from build123d import *

# Parameters (mm, degrees)
F0_W      = 20
F0_H      = 20
F1_DEPTH  = 20
F2_R      = 2.6
F3_DEPTH  = 1
F4_R      = 2.6
F5_DEPTH  = 1
F6_R      = 2.6
F7_DEPTH  = 1
F8_R      = 2.6
F9_DEPTH  = 1
F10_R     = 2.6
F11_DEPTH = 1
F13_DEPTH = 1


with BuildPart() as f1:
    # F0 (on Front) → F1 (new body)
    with BuildSketch(Plane.XZ):
        with Locations((10, 10)):
            Rectangle(F0_W, F0_H)
    extrude(amount=F1_DEPTH)

    # F2 (on face) → F3 (cut)
    with BuildSketch(Plane.XZ.offset(20)):
        with Locations((10, 10)):
            Circle(F2_R)
        with Locations((5, 15)):
            Circle(F2_R)
        with Locations((15, 15)):
            Circle(F2_R)
        with Locations((15, 5)):
            Circle(F2_R)
        with Locations((5, 5)):
            Circle(F2_R)
    extrude(amount=-F3_DEPTH, mode=Mode.SUBTRACT)

    # F4 (on face) → F5 (cut)
    with BuildSketch(Plane(origin=(0, 0, 0), x_dir=(-1, 0, 0), z_dir=(0, 1, 0))):
        with Locations((-5, 15)):
            Circle(F4_R)
        with Locations((-15, 5)):
            Circle(F4_R)
    extrude(amount=-F5_DEPTH, mode=Mode.SUBTRACT)

    # F6 (on face) → F7 (cut)
    with BuildSketch(Plane(origin=(0, 0, 0), x_dir=(0, -1, 0), z_dir=(-1, 0, 0))):
        with Locations((10, 10)):
            Circle(F6_R)
        with Locations((15, 15)):
            Circle(F6_R)
        with Locations((5, 5)):
            Circle(F6_R)
    extrude(amount=-F7_DEPTH, mode=Mode.SUBTRACT)

    # F8 (on face) → F9 (cut)
    with BuildSketch(Plane.YZ.offset(20)):
        with Locations((-15, 5)):
            Circle(F8_R)
        with Locations((-15, 15)):
            Circle(F8_R)
        with Locations((-5, 15)):
            Circle(F8_R)
        with Locations((-5, 5)):
            Circle(F8_R)
    extrude(amount=-F9_DEPTH, mode=Mode.SUBTRACT)

    # F10 (on face) → F11 (cut)
    with BuildSketch(Plane(origin=(0, 0, 0), x_dir=(1, 0, 0), z_dir=(0, 0, -1))):
        with Locations((10, 10)):
            Circle(F10_R)
    extrude(amount=-F11_DEPTH, mode=Mode.SUBTRACT)

    # F12 (on face) → F13 (cut)
    with BuildSketch(Plane.XY.offset(20)):
        with BuildLine():
            ThreePointArc((4, -6.6), (5.838478, -5.838478), (6.6, -4))
            ThreePointArc((6.6, -4), (5.838478, -2.161522), (4, -1.4))
            ThreePointArc((4, -1.4), (1.4, -4), (4, -6.6))
        make_face()
        with BuildLine():
            ThreePointArc((6.6, -16), (5.838478, -14.161522), (4, -13.4))
            ThreePointArc((4, -13.4), (2.161522, -14.161522), (1.4, -16))
            ThreePointArc((1.4, -16), (4, -18.6), (6.6, -16))
        make_face()
        with BuildLine():
            ThreePointArc((6.6, -10), (5.838478, -8.161522), (4, -7.4))
            ThreePointArc((4, -7.4), (1.4, -10), (4, -12.6))
            ThreePointArc((4, -12.6), (5.838478, -11.838478), (6.6, -10))
        make_face()
        with BuildLine():
            Line((13.4, -16), (18.6, -16))
            ThreePointArc((18.6, -16), (17.838478, -14.161522), (16, -13.4))
            ThreePointArc((16, -13.4), (14.161522, -14.161522), (13.4, -16))
        make_face()
        with BuildLine():
            ThreePointArc((13.4, -4), (14.161522, -5.838478), (16, -6.6))
            ThreePointArc((16, -6.6), (17.838478, -5.838478), (18.6, -4))
            Line((18.6, -4), (13.4, -4))
        make_face()
        with BuildLine():
            ThreePointArc((16, -7.4), (13.4, -10), (16, -12.6))
            ThreePointArc((16, -12.6), (17.838478, -11.838478), (18.6, -10))
            ThreePointArc((18.6, -10), (17.838478, -8.161522), (16, -7.4))
        make_face()
        with BuildLine():
            ThreePointArc((13.4, -16), (16, -18.6), (18.6, -16))
            Line((18.6, -16), (13.4, -16))
        make_face()
        with BuildLine():
            ThreePointArc((16, -1.4), (14.161522, -2.161522), (13.4, -4))
            Line((13.4, -4), (18.6, -4))
            ThreePointArc((18.6, -4), (17.838478, -2.161522), (16, -1.4))
        make_face()
    extrude(amount=-F13_DEPTH, mode=Mode.SUBTRACT)


solid = f1.part
For this review, take the finished solid that the model builds, in its own axes (mm). A direction names the side the tool comes from. Round coordinates to 2 decimals unless told otherwise and drop trailing zeros. Write each loop counter-clockwise with the first axis right and the second up, starting at its lowest first coordinate (ties: lowest second). Pieces come first, ordered by that corner, then holes. Notation, with made-up numbers: (18.25, 55.5) -> (25.25, 55.5) arc R8 cw to (25.25, 66.5) -> close; hole circle Ø8 at (64.25, 22). An arc over 180 degrees is marked (long way). Use CSV: the item, a comma, the result in double quotes.
(1) Clearance check with flat-ended pins moving along their axes: P1, Ø2.5, axis at x = 5, z = 14, coming from the +Y side; P2, Ø3, axis at y = -15, z = 14, coming from the +X side; P3, Ø3, axis at y = -15, z = 15, coming from the -X side. State where each tip first meets the part, or that it passes through.
Computed values:
P1,"y = -1"
P2,"x = 19"
P3,"x = 1"
(2) For faces 1 (the face through (16, -16, 19)), 2 (the face through (5, -19, 15)), 3 (the face through (0.493, -4.662, 7.578)), 4 (the face through (19, -15, 5)), list the 3-axis set-ups (+Z, -Z, +X, -X, +Y, -Y) from which the entire face can be reached by the end or side of a thin tool; tool diameter is ignored.
Computed values:
face 1,"+Z"
face 2,"-Y"
face 3,"-X"
face 4,"+X"
(3) Draft analysis for pull direction Y (two halves, no side actions). For faces 5 (the face through (3.8, -0.493, 12.693)), 6 (the face through (10, 0, 10)), 7 (the face through (19.51, -12.52, 5.78)), 8 (the face through (5, -19, 5)), state which applies: +Y half, -Y half, draft (parallel to the pull), parting line (faces both ways), or undercut.
Computed values:
face 5,"draft"
face 6,"+Y half"
face 7,"undercut"
face 8,"-Y half"
(4) Consider section D-D, the plane x = 10. Give the boundary of the cut face in (y, z).
Computed values:
outline,"(-20, 0) -> (-12.6, 0) -> (-12.6, 1) -> (-7.4, 1) -> (-7.4, 0) -> (0, 0) -> (0, 20) -> (-20, 20) -> (-20, 12.6) -> (-19, 12.6) -> (-19, 7.4) -> (-20, 7.4) -> close"
(5) To check wall thickness, follow L1, parallel to Z at x = 15, y = -0.55; L2, parallel to Z at x = 10, y = -19.25; L3, parallel to X at y = -9, z = 11.5. State the ranges of each line that lie inside material, in increasing order. Write a range as [from, to].
Computed values:
L1,"[0, 2.4], [7.6, 20]"
L2,"[0, 7.4], [12.6, 20]"
L3,"[1, 20]"
(6) Consider section B-B, the plane x = 15. Give the boundary of the cut face in (y, z).
Computed values:
outline,"(-20, 0) -> (0, 0) -> (0, 2.4) -> (-1, 2.4) -> (-1, 7.6) -> (0, 7.6) -> (0, 20) -> (-1.6, 20) -> (-1.6, 19) -> (-6.4, 19) -> (-6.4, 20) -> (-7.6, 20) -> (-7.6, 19) -> (-12.4, 19) -> (-12.4, 20) -> (-13.6, 20) -> (-13.6, 19) -> (-18.4, 19) -> (-18.4, 20) -> (-20, 20) -> (-20, 17.6) -> (-19, 17.6) -> (-19, 12.4) -> (-20, 12.4) -> (-20, 7.6) -> (-19, 7.6) -> (-19, 2.4) -> (-20, 2.4) -> close"
(7) Consider section C-C, the plane z = 10. Give the boundary of the cut face in (x, y).
Computed values:
outline,"(0, -20) -> (7.4, -20) -> (7.4, -19) -> (12.6, -19) -> (12.6, -20) -> (20, -20) -> (20, 0) -> (0, 0) -> (0, -7.4) -> (1, -7.4) -> (1, -12.6) -> (0, -12.6) -> close"
(8) Consider section A-A, the plane y = -5. Give the boundary of the cut face in (x, z).
Computed values:
outline,"(0, 0) -> (20, 0) -> (20, 2.4) -> (19, 2.4) -> (19, 7.6) -> (20, 7.6) -> (20, 12.4) -> (19, 12.4) -> (19, 17.6) -> (20, 17.6) -> (20, 20) -> (18.4, 20) -> (18.4, 19) -> (13.6, 19) -> (13.6, 20) -> (6.4, 20) -> (6.4, 19) -> (1.6, 19) -> (1.6, 20) -> (0, 20) -> (0, 7.6) -> (1, 7.6) -> (1, 2.4) -> (0, 2.4) -> close"
